The model under review builds one solid part; all positions refer to its coordinate system, in mm. Give positions to 0.01 mm unless a question says otherwise; leave off trailing zeros. Order: outer loops, then holes, each group sorted by start corner. A loop starts at its lowest first (then second) coordinate and runs counter-clockwise, first axis right, second up. Notation, with made-up numbers: (85.25, 83) - (130.25, 83) arc R24 ccw to (130.25, 94) - close; hole circle Ø7 at (37.5, 83.5). An arc over 180 degrees is marked (long way). Answer as CSV lines item,"result". Start each with the question number.
from build123d import *

# Parameters (mm, degrees)
F1_DEPTH = 3
F2_R     = 3
F3_R     = 1
F5_DEPTH = 25


with BuildPart() as f1:
    # F0 (on Top) → F1 (new body)
    with BuildSketch(Plane.XY):
        with BuildLine():
            ThreePointArc((-23.866491, -12.625), (6.504028, -26.204916), (27, 0))
            ThreePointArc((27, 0), (26.808472, 3.210273), (26.236604, 6.375))
            Line((26.236604, 6.375), (0, 6.375))
            ThreePointArc((0, 6.375), (-2.209709, 11.709709), (3.125, 9.5))
            Line((3.125, 9.5), (25.273504, 9.5))
            ThreePointArc((25.273504, 9.5), (-9.5, 25.273504), (-25.273504, -9.5))
            Line((-25.273504, -9.5), (-3.125, -9.5))
            ThreePointArc((-3.125, -9.5), (0, -6.375), (3.125, -9.5))
            ThreePointArc((3.125, -9.5), (2.209709, -11.709709), (0, -12.625))
            Line((0, -12.625), (-23.866491, -12.625))
        make_face()
    extrude(amount=F1_DEPTH)

    # F2
    f2_edges = [f1.edges().sort_by_distance(p)[0] for p in [
        (-25.273504, -9.5, 1.5),
        (26.236604, 6.375, 1.5),
    ]]
    fillet(f2_edges, radius=F2_R)

    # F3
    f3_edges = [f1.edges().sort_by_distance(p)[0] for p in [
        (25.273504, 9.5, 1.5),
        (-23.866491, -12.625, 1.5),
    ]]
    fillet(f3_edges, radius=F3_R)

    # F4 (on face) → F5 (cut)
    with BuildSketch(Plane.XY.offset(3)):
        with BuildLine():
            ThreePointArc((1.998628, 26.925926), (0, 27), (-1.998628, 26.925926))
            ThreePointArc((-1.998628, 26.925926), (0, 25), (1.998628, 26.925926))
        make_face()
        with BuildLine():
            ThreePointArc((-1.998628, -26.925926), (0, -27), (1.998628, -26.925926))
            ThreePointArc((1.998628, -26.925926), (0, -25), (-1.998628, -26.925926))
        make_face()
    extrude(amount=-F5_DEPTH, mode=Mode.SUBTRACT)


solid = f1.part
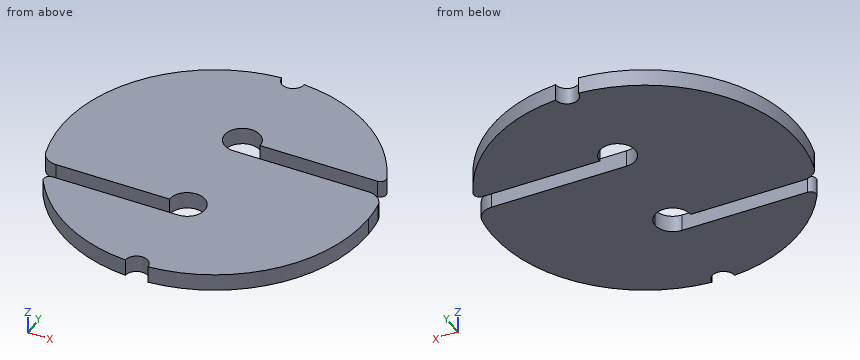
Item 1: Take a section at C-C on x = 10.5. Write out the cut boundary in (y, z) (3 decimals), and give its area (3 significant figures).
Item 2: For line 1 along Y through (x, z) = (0, 0.8) (3 decimals); line 2 along X through (y, z) = (-2, 0.9); line 3 along Y through (x, z) = (15.5, 1.4) (3 decimals), list the stretches that pass through material, from the lowest coordinate up.
Item 3: Take a section at D-D on y = -17. Write out the cut boundary in (x, z).
Item 4: Take a section at B-B on x = -17. Write out the cut boundary in (y, z) (3 decimals), and give its area (3 significant figures).
Item 5: Clearance check with flat-ended pins moving along their axes: pin 1 (1.5 mm diameter, centred on x = -14.5, z = 2, fed in from -Y); pin 2 (1.5 mm diameter, centred on x = -16.5, z = 1, fed in from +Y); pin 3 (1.5 mm diameter, centred on y = 7, z = 0.5, fed in from -X). State where each tip first meets the part, or that it passes through.
Data:
1,outline,"(-24.875, 0) - (6.375, 0) - (6.375, 3) - (-24.875, 3) - close; (9.5, 0) - (24.875, 0) - (24.875, 3) - (9.5, 3) - close"
1,area,"140 mm^2"
2,line 1,"y = -25 to -12.625, -6.375 to 6.375, 12.625 to 25"
2,line 2,"x = -26.93 to 26.93"
2,line 3,"y = -22.108 to 6.375, 9.5 to 22.108"
3,outline,"(-20.98, 0) - (20.98, 0) - (20.98, 3) - (-20.98, 3) - close"
4,outline,"(-20.976, 0) - (-12.625, 0) - (-12.625, 3) - (-20.976, 3) - close; (-9.5, 0) - (20.976, 0) - (20.976, 3) - (-9.5, 3) - close"
4,area,"116 mm^2"
5,pin 1,"stops at y = -23.24"
5,pin 2,"stops at y = 21.93"
5,pin 3,"stops at x = -26.27"
